The listing builds one solid part. Answer for the finished solid, in the listing's coordinates (mm). Give positions to 0.01 mm unless a question says otherwise; leave off trailing zeros. Write each loop counter-clockwise with the first axis right and the second up, starting at its lowest first coordinate (ties: lowest second). Pieces come first, ordered by that corner, then holes. Notation, with made-up numbers: (-12.75, -3.5) -> (33.25, -3.5) arc R12 cw to (33.25, 18.5) -> close; hole circle Ø6 at (22.25, -33). An arc over 180 degrees is marked (long way). Put each result on its own line as item: value. Start each with the question number.
1) A cutting plane is placed at D-D (x = -56.5). Write down the section's boundary in (y, z).
2) A cutting plane is placed at A-A (z = 2.75). Give the number of separate pieces and of enclosed holes in the cut face, then the cut area to 3 significant figures.
3) A cutting plane is placed at B-B (x = -43). Write down the section's boundary in (y, z).
4) Find the intervals of material crossed by line 1 along X through (y, z) = (54, 2); line 2 along Y through (x, z) = (0, 5); line 3 along X through (y, z) = (15, 3.75), in increasing order. Write a range as from..to.
5) Flat-ended cylindrical pins translate along their axes: pin 1 Ø1.5 at (y, z) = (-19.5, 5.5) entering from +X; pin 2 Ø0.9 at (y, z) = (-19.5, 6) entering from -X; pin 3 Ø1.5 at (x, z) = (18, 6) entering from -Y. Find the tip coordinate at first contact, or state that the pin passes through.
6) A cutting plane is placed at C-C (y = -47). Write down the section's boundary in (x, z), then the cut area to 3 significant figures.
from build123d import *

# Parameters (mm, degrees)
F0_R        = 1.25
F0_W        = 70
F0_H        = 60
F0_W_2      = 55
F0_H_2      = 35
F1_DEPTH    = 4
F2_DEPTH    = 7
F3_T1_DEPTH = 4
F3_T3_DEPTH = 50.3525491562
F3_T5_DEPTH = 98.5146090037
F3_T7_DEPTH = 40.5
F3_T9_DEPTH = 63.5146090037


# Not quite as in the source:
# - a fillet or chamfer that OpenCascade refuses, or shapes differently, is made with other operations: its cross-section is extruded or revolved along the edge and cut away or added


with BuildPart() as f1:
    # F0 (on Top) → F1 (new body)
    with BuildSketch(Plane.XY):
        Polygon((-40, 93.3383707737), (-70, 93.3383707737), (-35, -56.6616292263), (-35, 3.3383707737), (35, 3.3383707737), (35, -56.6616292263), (70, 93.3383707737), (40, 93.3383707737), (0, 13.3383707737), align=None)
        Polygon((-45.172164613, 13.3383707737), (-56.8388312797, 63.3383707737), (-31.7082039325, 63.3383707737), (-6.7082039325, 13.3383707737), align=None, mode=Mode.SUBTRACT)
        with Locations((-50, 78.3383707737)):
            Circle(F0_R, mode=Mode.SUBTRACT)
        Polygon((6.7082039325, 13.3383707737), (31.7082039325, 63.3383707737), (56.8388312797, 63.3383707737), (45.172164613, 13.3383707737), align=None, mode=Mode.SUBTRACT)
        with Locations((50, 78.3383707737)):
            Circle(F0_R, mode=Mode.SUBTRACT)
        with Locations((0, -26.6616292263)):
            Rectangle(F0_W, F0_H)
        with Locations((0, -19.1616292263)):
            Rectangle(F0_W_2, F0_H_2, mode=Mode.SUBTRACT)
        with Locations((0, -19.1616292263)):
            Rectangle(F0_W_2, F0_H_2)
        with Locations((-10, -19.1616292263)):
            Circle(F0_R, mode=Mode.SUBTRACT)
        with Locations((0, -19.1616292263)):
            Circle(F0_R, mode=Mode.SUBTRACT)
        with Locations((10, -19.1616292263)):
            Circle(F0_R, mode=Mode.SUBTRACT)
    extrude(amount=F1_DEPTH)

    # F0 (on Top) → F2 (join)
    with BuildSketch(Plane.XY):
        with Locations((0, -19.1616292263)):
            Rectangle(F0_W_2, F0_H_2)
        with Locations((-10, -19.1616292263)):
            Circle(F0_R, mode=Mode.SUBTRACT)
        with Locations((0, -19.1616292263)):
            Circle(F0_R, mode=Mode.SUBTRACT)
        with Locations((10, -19.1616292263)):
            Circle(F0_R, mode=Mode.SUBTRACT)
    extrude(amount=F2_DEPTH)

    # F3: fillet of radius 15 on 19 edges, made by hand

    # F3_s2 → F3_t1 (join)
    with BuildSketch(Plane.XY):
        with BuildLine():
            ThreePointArc((13.416407865, 40.1711865037), (0, 31.8793904362), (-13.416407865, 40.1711865037))
            Line((-13.416407865, 40.1711865037), (0, 13.3383707737))
            Line((0, 13.3383707737), (13.416407865, 40.1711865037))
        make_face()
        with BuildLine():
            ThreePointArc((17.5623058987, 35.0465747062), (18.2189516385, 20.452404092), (30.9787137637, 13.3383707737))
            Line((30.9787137637, 13.3383707737), (6.7082039325, 13.3383707737))
            Line((6.7082039325, 13.3383707737), (17.5623058987, 35.0465747062))
        make_face()
        with BuildLine():
            ThreePointArc((47.8768609584, 24.9299265396), (42.5932263089, 16.5883353799), (33.2692428123, 13.3383707737))
            Line((33.2692428123, 13.3383707737), (45.172164613, 13.3383707737))
            Line((45.172164613, 13.3383707737), (47.8768609584, 24.9299265396))
        make_face()
        with BuildLine():
            ThreePointArc((-17.5623058987, 35.0465747062), (-18.2189516385, 20.452404092), (-30.9787137637, 13.3383707737))
            Line((-30.9787137637, 13.3383707737), (-6.7082039325, 13.3383707737))
            Line((-6.7082039325, 13.3383707737), (-17.5623058987, 35.0465747062))
        make_face()
        with BuildLine():
            ThreePointArc((-47.8768609584, 24.9299265396), (-42.5932263089, 16.5883353799), (-33.2692428123, 13.3383707737))
            Line((-33.2692428123, 13.3383707737), (-45.172164613, 13.3383707737))
            Line((-45.172164613, 13.3383707737), (-47.8768609584, 24.9299265396))
        make_face()
        with BuildLine():
            ThreePointArc((-37.935909479, 63.3383707737), (-49.6859448728, 57.6623542703), (-52.5435276251, 44.9299265396))
            Line((-52.5435276251, 44.9299265396), (-56.8388312797, 63.3383707737))
            Line((-56.8388312797, 63.3383707737), (-37.935909479, 63.3383707737))
        make_face()
        with BuildLine():
            ThreePointArc((-40.9787137637, 63.3383707737), (-33.092747082, 61.098132899), (-27.5623058987, 55.0465747062))
            Line((-27.5623058987, 55.0465747062), (-31.7082039325, 63.3383707737))
            Line((-31.7082039325, 63.3383707737), (-40.9787137637, 63.3383707737))
        make_face()
        with BuildLine():
            ThreePointArc((40.9787137637, 63.3383707737), (33.092747082, 61.098132899), (27.5623058987, 55.0465747062))
            Line((27.5623058987, 55.0465747062), (31.7082039325, 63.3383707737))
            Line((31.7082039325, 63.3383707737), (40.9787137637, 63.3383707737))
        make_face()
        with BuildLine():
            ThreePointArc((37.935909479, 63.3383707737), (49.6859448728, 57.6623542703), (52.5435276251, 44.9299265396))
            Line((52.5435276251, 44.9299265396), (56.8388312797, 63.3383707737))
            Line((56.8388312797, 63.3383707737), (37.935909479, 63.3383707737))
        make_face()
    extrude(amount=F3_T1_DEPTH)

    # F3_s4 → F3_t3 (cut)
    with BuildSketch(Plane.XY.offset(-23.1762745781)):
        with BuildLine():
            ThreePointArc((49.2705098312, 93.3383707737), (41.3845431495, 91.098132899), (35.8541019662, 85.0465747062))
            Line((35.8541019662, 85.0465747062), (40, 93.3383707737))
            Line((40, 93.3383707737), (49.2705098312, 93.3383707737))
        make_face()
        with BuildLine():
            ThreePointArc((-49.2705098312, 93.3383707737), (-41.3845431495, 91.098132899), (-35.8541019662, 85.0465747062))
            Line((-35.8541019662, 85.0465747062), (-40, 93.3383707737))
            Line((-40, 93.3383707737), (-49.2705098312, 93.3383707737))
        make_face()
    extrude(amount=F3_T3_DEPTH, mode=Mode.SUBTRACT)

    # F3_s6 → F3_t5 (cut)
    with BuildSketch(Plane.XY.offset(-47.2573045019)):
        with BuildLine():
            ThreePointArc((65.7046963454, 74.9299265396), (62.8471135931, 87.6623542703), (51.0970781993, 93.3383707737))
            Line((51.0970781993, 93.3383707737), (70, 93.3383707737))
            Line((70, 93.3383707737), (65.7046963454, 74.9299265396))
        make_face()
        with BuildLine():
            ThreePointArc((-51.0970781993, 93.3383707737), (-62.8471135931, 87.6623542703), (-65.7046963454, 74.9299265396))
            Line((-65.7046963454, 74.9299265396), (-70, 93.3383707737))
            Line((-70, 93.3383707737), (-51.0970781993, 93.3383707737))
        make_face()
    extrude(amount=F3_T5_DEPTH, mode=Mode.SUBTRACT)

    # F3_s8 → F3_t7 (cut)
    with BuildSketch(Plane.XY.offset(4)):
        with BuildLine():
            ThreePointArc((12.5, -1.6616292263), (23.1066017178, -6.0550275085), (27.5, -16.6616292263))
            Line((27.5, -16.6616292263), (27.5, -1.6616292263))
            Line((27.5, -1.6616292263), (12.5, -1.6616292263))
        make_face()
        with BuildLine():
            ThreePointArc((-12.5, -1.6616292263), (-23.1066017178, -6.0550275085), (-27.5, -16.6616292263))
            Line((-27.5, -16.6616292263), (-27.5, -1.6616292263))
            Line((-27.5, -1.6616292263), (-12.5, -1.6616292263))
        make_face()
        with BuildLine():
            ThreePointArc((12.5, -36.6616292263), (23.1066017178, -32.2682309441), (27.5, -21.6616292263))
            Line((27.5, -21.6616292263), (27.5, -36.6616292263))
            Line((27.5, -36.6616292263), (12.5, -36.6616292263))
        make_face()
        with BuildLine():
            ThreePointArc((-27.5, -21.6616292263), (-23.1066017178, -32.2682309441), (-12.5, -36.6616292263))
            Line((-12.5, -36.6616292263), (-27.5, -36.6616292263))
            Line((-27.5, -36.6616292263), (-27.5, -21.6616292263))
        make_face()
    extrude(amount=F3_T7_DEPTH, mode=Mode.SUBTRACT)

    # F3_s10 → F3_t9 (cut)
    with BuildSketch(Plane.XY.offset(-29.7573045019)):
        with BuildLine():
            ThreePointArc((-37.7046963454, -45.0700734604), (-32.4210616958, -53.4116646201), (-23.0970781993, -56.6616292263))
            Line((-23.0970781993, -56.6616292263), (-35, -56.6616292263))
            Line((-35, -56.6616292263), (-37.7046963454, -45.0700734604))
        make_face()
        with BuildLine():
            ThreePointArc((23.0970781993, -56.6616292263), (32.4210616958, -53.4116646201), (37.7046963454, -45.0700734604))
            Line((37.7046963454, -45.0700734604), (35, -56.6616292263))
            Line((35, -56.6616292263), (23.0970781993, -56.6616292263))
        make_face()
    extrude(amount=F3_T9_DEPTH, mode=Mode.SUBTRACT)


solid = f1.part
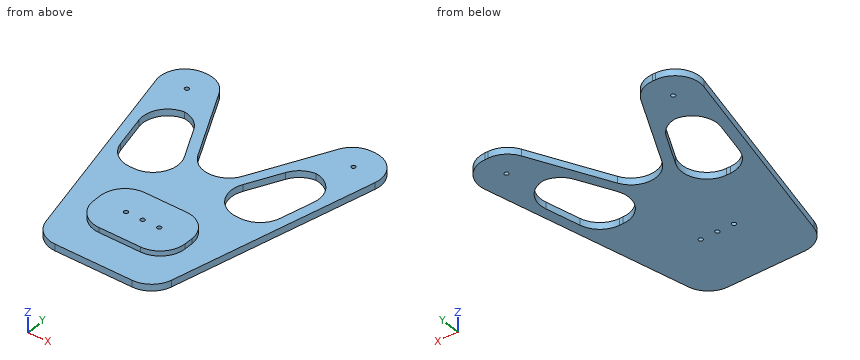
Reply:
1. outline: (35.48, 0) -> (92.33, 0) -> (92.33, 4) -> (35.48, 4) -> close
2. separate pieces: 1
2. enclosed holes: 7
2. area: 9,820 mm2
3. outline: (-22.38, 0) -> (16.92, 0) -> (16.92, 4) -> (-22.38, 4) -> close; (62.46, 0) -> (91.96, 0) -> (91.96, 4) -> (62.46, 4) -> close
4. line 1: x = -60.82..-51.83, -27.04..-20.33, 20.33..27.04, 51.83..60.82
4. line 2: y = -36.66..-20.41, -17.91..-1.66
4. line 3: x = -51.72..-40.13, -24.12..24.12, 40.13..51.72
5. pin 1: stops at x = 27.5
5. pin 2: stops at x = -27.5
5. pin 3: stops at y = -35.89
6. outline: (-37.11, 0) -> (37.11, 0) -> (37.11, 4) -> (-37.11, 4) -> close
6. area: 297 mm2
